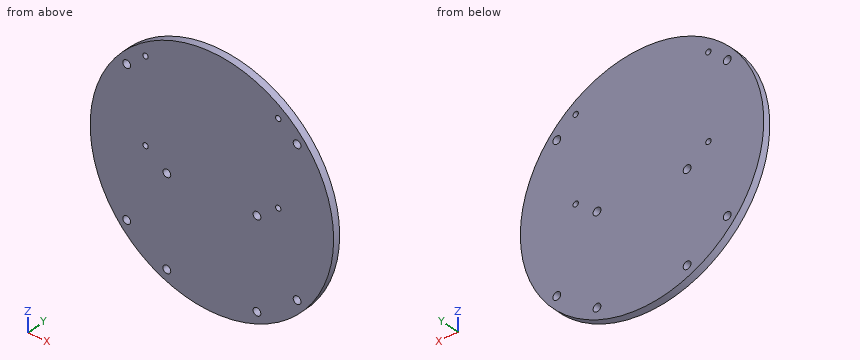
```python
from build123d import *

# Parameters (mm, degrees)
SKETCH1_R           = 50
SKETCH1_R_2         = 1.1
SKETCH1_R_3         = 1.6
BOSS_EXTRUDE1_DEPTH = 3


with BuildPart() as part:
    # Sketch1 → Boss-Extrude1 (new body)
    with BuildSketch(Plane(origin=(0, 0, 0), x_dir=(1, 0, 0), z_dir=(0, 1, 0))):
        Circle(SKETCH1_R)
        with Locations((-27.25, -2)):
            Circle(SKETCH1_R_2, mode=Mode.SUBTRACT)
        with Locations((-27.25, -36.5)):
            Circle(SKETCH1_R_2, mode=Mode.SUBTRACT)
        with Locations((27.25, -2)):
            Circle(SKETCH1_R_2, mode=Mode.SUBTRACT)
        with Locations((27.25, -36.5)):
            Circle(SKETCH1_R_2, mode=Mode.SUBTRACT)
        with Locations((-18.5, 41.75)):
            Circle(SKETCH1_R_3, mode=Mode.SUBTRACT)
        with Locations((18.5, 41.75)):
            Circle(SKETCH1_R_3, mode=Mode.SUBTRACT)
        with Locations((18.5, 4.75)):
            Circle(SKETCH1_R_3, mode=Mode.SUBTRACT)
        with Locations((-18.5, 4.75)):
            Circle(SKETCH1_R_3, mode=Mode.SUBTRACT)
        with Locations((-35, -30)):
            Circle(SKETCH1_R_3, mode=Mode.SUBTRACT)
        with Locations((-35, 30)):
            Circle(SKETCH1_R_3, mode=Mode.SUBTRACT)
        with Locations((35, -30)):
            Circle(SKETCH1_R_3, mode=Mode.SUBTRACT)
        with Locations((35, 30)):
            Circle(SKETCH1_R_3, mode=Mode.SUBTRACT)
    extrude(amount=BOSS_EXTRUDE1_DEPTH)


solid = part.part
```
Work out the finished part from the listing and answer in its coordinate system (mm). Give positions to 0.01 mm unless a question says otherwise; leave off trailing zeros. Write each loop counter-clockwise with the first axis right and the second up, starting at its lowest first coordinate (ties: lowest second). Pieces come first, ordered by that corner, then holes. Notation, with made-up numbers: (57, 10.25) -> (88, 10.25) arc R14 ccw to (88, 22.25) -> close; hole circle Ø6 at (-19.75, 53.5). An arc over 180 degrees is marked (long way). Write each question's results on one line, items separated by ' | '.
1. Find section C-C on y = 1.65. Give the number of separate pieces and of enclosed holes in the cut face, and give its area (3 significant figures).
Data:
separate pieces: 1 | enclosed holes: 12 | area: 7,770 mm^2
2. Find section A-A on z = -30. Determine the outline of the cut face in (x, y), and give its area (3 significant figures).
Data:
outline: (-40, 0) -> (-36.6, 0) -> (-36.6, 3) -> (-40, 3) -> close; (-33.4, 0) -> (33.4, 0) -> (33.4, 3) -> (-33.4, 3) -> close; (36.6, 0) -> (40, 0) -> (40, 3) -> (36.6, 3) -> close | area: 221 mm^2
3. Find section D-D on z = 20.5. Determine the outline of the cut face in (x, y).
Data:
outline: (-45.6, 0) -> (45.6, 0) -> (45.6, 3) -> (-45.6, 3) -> close
4. Straight lines are drawn through the part: L1, parallel to Z at x = 35, y = 1.25; L2, parallel to Z at x = -18.5, y = 2.3; L3, parallel to X at y = 0.6, z = 36.5. For each, find the intervals that lie inside material, in ascending order.
Data:
L1: -35.71 to -31.6, -28.4 to 28.4, 31.6 to 35.71 | L2: -46.45 to -43.35, -40.15 to -6.35, -3.15 to 46.45 | L3: -34.17 to -28.35, -26.15 to 26.15, 28.35 to 34.17
5. Find section B-B on x = 35. Determine the outline of the cut face in (y, z).
Data:
outline: (0, -35.71) -> (3, -35.71) -> (3, -31.6) -> (0, -31.6) -> close; (0, -28.4) -> (3, -28.4) -> (3, 28.4) -> (0, 28.4) -> close; (0, 31.6) -> (3, 31.6) -> (3, 35.71) -> (0, 35.71) -> close
6. Each of these flat-tipped pins is pushed along its axis until it touches: pin 1 Ø1.5 at (x, y) = (-9, 0.5) entering from -Z; pin 2 Ø5 at (x, z) = (35, 30) entering from -Y. Where does it stop, or does it pass through?
Data:
pin 1: z = -49.31 | pin 2: y = 0
